Part print with two shaded views. Sizes in mm from the minimum x, y, z corner. A direction names the side the tool comes from. Give positions to 0.01 mm unless a question says otherwise; leave off trailing zeros. Write each loop counter-clockwise with the first axis right and the second up, starting at its lowest first coordinate (ties: lowest second). Pieces come first, ordered by that corner, then holes.
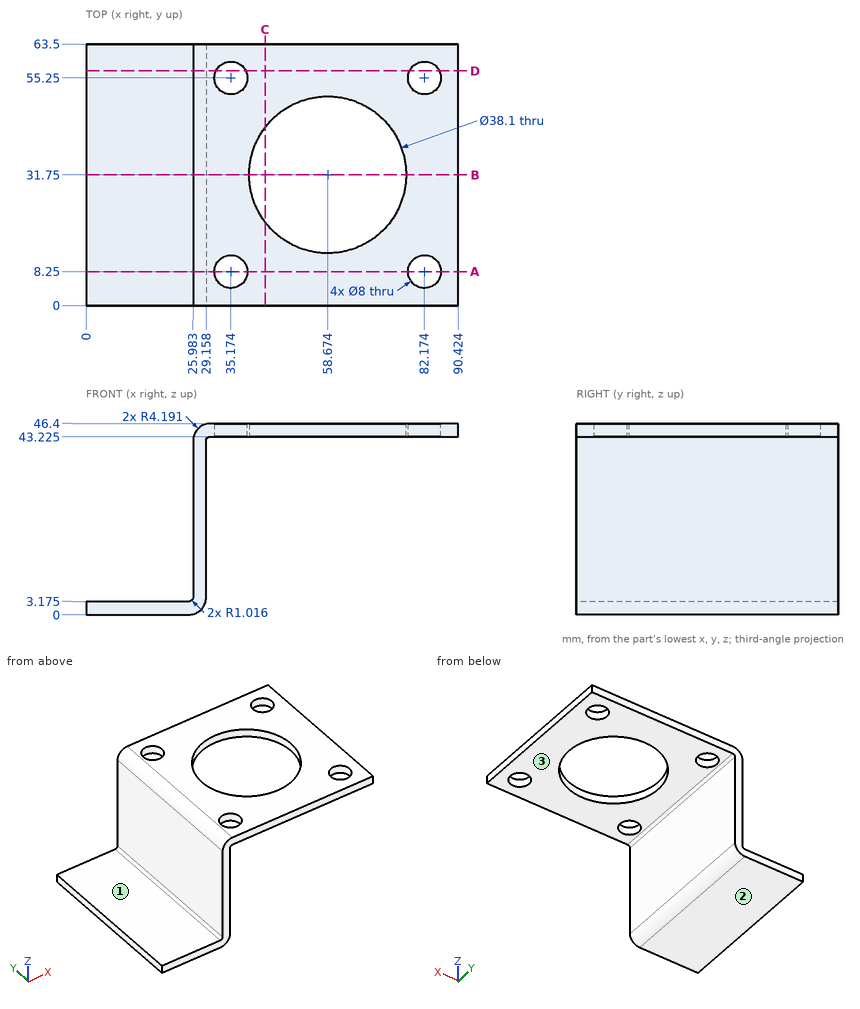
(1) 3-axis set-ups, long thin cutter, end or side, ignore diameter. For the marked faces 1, 2 and 3: which of +Z, -Z, +X, -X, +Y, -Y reach the whole face in a straight line?
(2) Drop flat-ended pins along their axis: pin 1 (6 mm diameter, centred on y = 24, z = 25.5, fed in from +X); pin 2 (19 mm diameter, centred on y = 29.5, z = 32.5, fed in from -X); pin 3 (9 mm diameter, centred on x = 35.17, y = 55.25, fed in from -Z) (3 decimals). Give the stop position or say it passes through.
(3) Saw through at D-D, the plane y = 57. List the corners of the cut face in (x, z) (1 decimal).
(4) Probe line 1 (X direction, y = 55.25, z = 45.4); line 2 (X direction, y = 8.25, z = 45.05); line 3 (X direction, y = 59, z = 13). List the from-to ranges inside material, lowest first.
(5) Saw through at A-A, the plane y = 8.25. List the corners of the cut face in (x, z) (3 decimals).
(6) Saw through at C-C, the plane x = 43.5. List the corners of the cut face in (y, z) (1 decimal), plus the area to 3 significant figures.
(7) Saw through at B-B, the plane y = 31.75. List the corners of the cut face in (x, z) (3 decimals).
Computed values:
1. face 1: +Z, -X, +Y, -Y
1. face 2: -Z, +X, -X, +Y, -Y
1. face 3: -Z, +X, +Y, -Y
2. pin 1: stops at x = 29.16
2. pin 2: stops at x = 25.98
2. pin 3: stops at z = 43.225
3. outline: (0, 0) - (25, 0) arc R4.2 ccw to (29.2, 4.2) - (29.2, 42.2) arc R1 cw to (30.2, 43.2) - (31.6, 43.2) - (31.6, 46.4) - (30.2, 46.4) arc R4.2 ccw to (26, 42.2) - (26, 4.2) arc R1 cw to (25, 3.2) - (0, 3.2) - close; (38.8, 43.2) - (78.6, 43.2) - (78.6, 46.4) - (38.8, 46.4) - close; (85.8, 43.2) - (90.4, 43.2) - (90.4, 46.4) - (85.8, 46.4) - close
4. line 1: x = 27.46 to 31.17, 39.17 to 78.17, 86.17 to 90.42
4. line 2: x = 27.09 to 31.17, 39.17 to 78.17, 86.17 to 90.42
4. line 3: x = 25.98 to 29.16
5. outline: (0, 0) - (24.967, 0) arc R4.191 ccw to (29.158, 4.191) - (29.158, 42.209) arc R1.016 cw to (30.174, 43.225) - (31.174, 43.225) - (31.174, 46.4) - (30.174, 46.4) arc R4.191 ccw to (25.983, 42.209) - (25.983, 4.191) arc R1.016 cw to (24.967, 3.175) - (0, 3.175) - close; (39.174, 43.225) - (78.174, 43.225) - (78.174, 46.4) - (39.174, 46.4) - close; (86.174, 43.225) - (90.424, 43.225) - (90.424, 46.4) - (86.174, 46.4) - close
6. outline: (0, 43.2) - (20.2, 43.2) - (20.2, 46.4) - (0, 46.4) - close; (43.3, 43.2) - (63.5, 43.2) - (63.5, 46.4) - (43.3, 46.4) - close
6. area: 128 mm2
7. outline: (0, 0) - (24.967, 0) arc R4.191 ccw to (29.158, 4.191) - (29.158, 42.209) arc R1.016 cw to (30.174, 43.225) - (39.624, 43.225) - (39.624, 46.4) - (30.174, 46.4) arc R4.191 ccw to (25.983, 42.209) - (25.983, 4.191) arc R1.016 cw to (24.967, 3.175) - (0, 3.175) - close; (77.724, 43.225) - (90.424, 43.225) - (90.424, 46.4) - (77.724, 46.4) - close
